Geometry check sheet. Reference: the model listing, model coordinates, mm. Face numbers are marked on the shaded views. A direction names the side the tool comes from. Give positions to 0.01 mm unless a question says otherwise; leave off trailing zeros. Write each loop counter-clockwise with the first axis right and the second up, starting at its lowest first coordinate (ties: lowest second). Pieces come first, ordered by that corner, then holes. Notation, with made-up numbers: (-17.5, 62.5) - (2.5, 62.5) arc R14 ccw to (2.5, 82.5) - close; hole circle Ø9 at (44, 7). An arc over 180 degrees is marked (long way). Write item = value, one per line. Start each with the question number.
(1) Section check A-A, the plane x = 33. Enter the section's corners in (y, z).
(2) Section check C-C, the plane x = 0. Enter the section's corners in (y, z).
(3) Section check B-B, the plane z = -29.5. Enter the section's corners in (x, y), plus the area to 3 significant figures.
(4) Thickness scan on L1, parallel to Y at x = 0, z = -8.5; L2, parallel to Z at x = 117.5, y = 0; L3, parallel to Y at x = -14, z = -9. Record the ranges inside material, lowest first.
(5) Depth check by flat-ended pin: pin 1 Ø6 at (x, z) = (-40, -3.5) entering from -Y; pin 2 Ø1 at (y, z) = (-9, -5) entering from +X; pin 3 Ø25 at (y, z) = (4, 9) entering from +X; pin 4 Ø1 at (x, z) = (-42.5, -26) entering from +Y. Enter the tip coordinate at first touch or a pass-through.
(6) Access from +Z, -Z, +X, -X, +Y, -Y to the whole of each face (thin tool, end or side, straight path). Record for the marked faces 1 and 2.
(7) Section check D-D, the plane x = 83. Enter the section's corners in (y, z).
(8) Draft check along Y on the marked faces 3, 4 and 5. Enter one of: pulls with the +Y half, pulls with the -Y half, needs draft (parallel to the pull), parting line crosses it, or undercut.
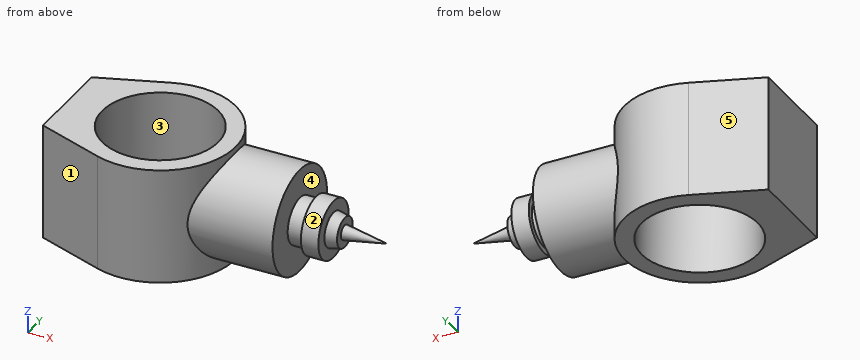
```python
from build123d import *

# Parameters (mm, degrees)
SKETCH1_R           = 50
BOSS_EXTRUDE1_DEPTH = 50
BOSS_EXTRUDE2_REACH = 202
SKETCH2_R           = 45


with BuildPart() as part:
    # Sketch1 → Boss-Extrude1 (new body, symmetric)
    with BuildSketch(Plane.XY):
        with BuildLine():
            Line((-80, 40), (-80, -40))
            Line((-80, -40), (-22.281665693, -61.061668614))
            ThreePointArc((-22.281665693, -61.061668614), (65, 0), (-22.281665693, 61.061668614))
            Line((-22.281665693, 61.061668614), (-80, 40))
        make_face()
        Circle(SKETCH1_R, mode=Mode.SUBTRACT)
    extrude(amount=BOSS_EXTRUDE1_DEPTH, both=True)

    # Sketch2 → Boss-Extrude2 (add, up to next)
    with BuildSketch(Plane(origin=(120, 0, 0), x_dir=(0, 0, -1), z_dir=(1, 0, 0)), mode=Mode.PRIVATE) as boss_extrude2_sk1:
        Circle(SKETCH2_R)
    boss_extrude2_tool1 = extrude(boss_extrude2_sk1.sketch, amount=-BOSS_EXTRUDE2_REACH, mode=Mode.PRIVATE) - part.part
    add(boss_extrude2_tool1.solids().sort_by_distance((120, 0, 0))[0])

    # Sketch4 → Revolve1 (revolve)
    with BuildSketch(Plane.XY):
        Polygon((120, -20), (134, -20), (134, -25), (149, -25), (149, -15), (158.789932038, -12.961071192), (158.529899955, -6.239535459), (195, 0), (120, 0), align=None)
    revolve(axis=Axis((120, 0, 0), (1, 0, 0)))


solid = part.part
```
Model answer:
q1.outline = (-56, -50) - (-37.56, -50) - (-37.56, 50) - (-56, 50) - close; (37.56, -50) - (56, -50) - (56, 50) - (37.56, 50) - close
q2.outline = (-65, -50) - (-50, -50) - (-50, 50) - (-65, 50) - close; (50, -50) - (65, -50) - (65, 50) - (50, 50) - close
q3.outline = (-80, -40) - (-22.28, -61.06) arc R65 ccw to (55.41, -33.98) - (120, -33.98) - (120, 33.98) - (55.41, 33.98) arc R65 ccw to (-22.28, 61.06) - (-80, 40) - close; hole circle Ø100 at (0, 0)
q3.area = 11,400 mm²
q4.L1 = -65 to -50, 50 to 65
q4.L2 = -45 to 45
q4.L3 = -63.47 to -48, 48 to 63.47
q5.pin_1 = -55.69
q5.pin_2 = 158.71
q5.pin_3 = 195
q5.pin_4 = 53.87
q6.face_1 = +Z, -Z, -X, -Y
q6.face_2 = +X
q7.outline = circle Ø90 at (0, 0)
q8.face_3 = undercut
q8.face_4 = needs draft
q8.face_5 = pulls with the +Y half
